Part model, mm, in its own coordinate system. Face numbers are marked on the shaded views. A direction names the side the tool comes from. Coordinates: 2 decimals unless noted, no trailing zeros. Order: outer loops, then holes, each group sorted by start corner. A loop starts at its lowest first (then second) coordinate and runs counter-clockwise, first axis right, second up. Notation, with made-up numbers: (6, -17) - (28, -17) arc R21 ccw to (28, 22) - close; hole circle Ø2 at (18.5, 36). An arc over 180 degrees is marked (long way). Use a Markdown table: item, result. Add a question column.
1) Tool access for the marked faces 1, 2 and 3: list every direction of +Z, -Z, +X, -X, +Y, -Y with a clear straight run to the whole face (end or side of a thin tool).
2) Two-plate mould, pull along X, no slides. Class the marked faces 4, 5 and 6: +X half, -X half, draft (parallel to the pull), parting line (faces both ways), or undercut.
3) Saw through at B-B on x = -22. List the corners of the cut face in (y, z).
4) Drop flat-ended pins along their axis: P1, Ø3, axis at y = 3.5, z = -4, coming from the -X side; P2, Ø3, axis at x = -11.5, y = -0.5, coming from the +Z side; P3, Ø2.5, axis at x = -25, z = -0.5, coming from the +Y side; P4, Ø4, axis at x = -17.5, y = 1, coming from the -Z side. Give the stop position or say it passes through.
5) Saw through at A-A on x = -11.5. List the corners of the cut face in (y, z).
6) Wall check: L1, parallel to X at y = -1, z = -6.5; L2, parallel to Y at x = -14, z = -8.25; L3, parallel to Y at x = -20.25, z = -9. Give the ranges that are in metal, low to high. Write a range as [from, to].
```python
from build123d import *
from build123d.topology import SkipClean

# Parameters (mm, degrees)
BOSS_EXTRUDE1_DEPTH = 1
CUT_EXTRUDE1_DEPTH  = 0.5
BOSS_EXTRUDE2_START = -25
BOSS_EXTRUDE2_DEPTH = 25
BOSS_EXTRUDE3_START = 1
BOSS_EXTRUDE3_DEPTH = 1
SKETCH7_R           = 0.5
BOSS_EXTRUDE4_DEPTH = 22.5
SKETCH10_R          = 0.5
CUT_EXTRUDE4_DEPTH  = 40.5
SKETCH8_W           = 10.868003522
SKETCH8_H           = 5.625
CUT_EXTRUDE2_DEPTH  = 22.5
LPATTERN1_COUNT     = 2
LPATTERN1_PITCH     = 11.25
CUT_EXTRUDE3_START  = -40.5
SKETCH9_R           = 20.473718745
SKETCH9_R_2         = 11.25
CUT_EXTRUDE3_DEPTH  = 40.5
SKETCH11_W          = 6.72531589
SKETCH11_H          = 3.584111804
SKETCH11_W_2        = 7.229090256
SKETCH11_H_2        = 3.619498095
CUT_EXTRUDE5_DEPTH  = 40.5
FILLET1_R           = 3


with BuildPart() as part:
    # Sketch1 → Boss-Extrude1 (new body)
    with BuildSketch(Plane(origin=(0, 0, 0), x_dir=(0, 0, -1), z_dir=(1, 0, 0))):
        with BuildLine():
            Line((0, -2.25), (0, -10.25))
            ThreePointArc((0, -10.25), (10.25, 0), (0, 10.25))
            Line((0, 10.25), (0, 2.25))
            ThreePointArc((0, 2.25), (1.590990258, 1.590990258), (2.25, 0))
            ThreePointArc((2.25, 0), (1.590990258, -1.590990258), (0, -2.25))
        make_face()
    extrude(amount=BOSS_EXTRUDE1_DEPTH)

    # Sketch2 → Cut-Extrude1 (cut)
    with BuildSketch(Plane.ZY):
        with BuildLine():
            ThreePointArc((0, 3.75), (2.651650429, 2.651650429), (3.75, 0))
            ThreePointArc((3.75, 0), (2.651650429, -2.651650429), (0, -3.75))
            Line((0, -3.75), (0, -4.75))
            ThreePointArc((0, -4.75), (3.358757211, -3.358757211), (4.75, 0))
            ThreePointArc((4.75, 0), (3.358757211, 3.358757211), (0, 4.75))
            Line((0, 4.75), (0, 3.75))
        make_face()
        with BuildLine():
            ThreePointArc((0, -3.75), (-3.75, 0), (0, 3.75))
            Line((0, 3.75), (0, 4.75))
            ThreePointArc((0, 4.75), (-4.75, 0), (0, -4.75))
            Line((0, -4.75), (0, -3.75))
        make_face()
        with BuildLine():
            Line((0, 6.75), (0, 5.75))
            ThreePointArc((0, 5.75), (4.065863992, 4.065863992), (5.75, 0))
            ThreePointArc((5.75, 0), (4.065863992, -4.065863992), (0, -5.75))
            Line((0, -5.75), (0, -6.75))
            ThreePointArc((0, -6.75), (4.772970773, -4.772970773), (6.75, 0))
            ThreePointArc((6.75, 0), (4.772970773, 4.772970773), (0, 6.75))
        make_face()
        with BuildLine():
            ThreePointArc((0, -5.75), (-5.75, 0), (0, 5.75))
            Line((0, 5.75), (0, 6.75))
            ThreePointArc((0, 6.75), (-6.75, 0), (0, -6.75))
            Line((0, -6.75), (0, -5.75))
        make_face()
        with BuildLine():
            Line((0, 8.75), (0, 7.75))
            ThreePointArc((0, 7.75), (5.480077554, 5.480077554), (7.75, 0))
            ThreePointArc((7.75, 0), (5.480077554, -5.480077554), (0, -7.75))
            Line((0, -7.75), (0, -8.75))
            ThreePointArc((0, -8.75), (6.187184335, -6.187184335), (8.75, 0))
            ThreePointArc((8.75, 0), (6.187184335, 6.187184335), (0, 8.75))
        make_face()
        with BuildLine():
            ThreePointArc((0, -7.75), (-7.75, 0), (0, 7.75))
            Line((0, 7.75), (0, 8.75))
            ThreePointArc((0, 8.75), (-8.75, 0), (0, -8.75))
            Line((0, -8.75), (0, -7.75))
        make_face()
    extrude(amount=-CUT_EXTRUDE1_DEPTH, mode=Mode.SUBTRACT)

    # Sketch3 → Boss-Extrude2 (add)
    with BuildSketch(Plane(origin=(1, 0, 0), x_dir=(0, 0, -1), z_dir=(1, 0, 0)).offset(BOSS_EXTRUDE2_START)):
        with BuildLine():
            Line((0, -10.25), (0, -11.25))
            ThreePointArc((0, -11.25), (11.25, 0), (0, 11.25))
            Line((0, 11.25), (0, 10.25))
            ThreePointArc((0, 10.25), (10.25, 0), (0, -10.25))
        make_face()
    extrude(amount=BOSS_EXTRUDE2_DEPTH)

    # Sketch6 → Boss-Extrude3 (add)
    with BuildSketch(Plane.ZY.offset(24).offset(BOSS_EXTRUDE3_START)):
        with BuildLine():
            Line((0, 11.25), (0, -11.25))
            ThreePointArc((0, -11.25), (-11.25, 0), (0, 11.25))
        make_face()
    extrude(amount=-BOSS_EXTRUDE3_DEPTH)

    # Sketch7 → Boss-Extrude4 (add)
    with SkipClean():  # the faces are left unmerged after this step: merging them gives an invalid solid
        with BuildSketch(Plane(origin=(0, 11.25, 0), x_dir=(1, 0, 0), z_dir=(0, 1, 0))):
            with BuildLine():
                Line((-23.585786438, 0), (-25, 1.414213562))
                Line((-25, 1.414213562), (-25.707106781, 0.707106781))
                ThreePointArc((-25.707106781, 0.707106781), (-25.707106781, -0.707106781), (-24.292893219, -0.707106781))
                Line((-24.292893219, -0.707106781), (-23.585786438, 0))
            make_face()
            with Locations(Location((-25, 0, 0), (0, 0, 270))):
                Circle(SKETCH7_R, mode=Mode.SUBTRACT)
        extrude(amount=-BOSS_EXTRUDE4_DEPTH)

    # Sketch10 → Cut-Extrude4 (cut)
    with BuildSketch(Plane(origin=(0, 11.25, 0), x_dir=(1, 0, 0), z_dir=(0, 1, 0))):
        with Locations(Location((-25, 0, 0), (0, 0, 270))):
            Circle(SKETCH10_R)
    extrude(amount=-CUT_EXTRUDE4_DEPTH, mode=Mode.SUBTRACT)

    # Sketch8 → Cut-Extrude2 (cut)
    with BuildSketch(Plane(origin=(-11.792893219, 0, -11.792893219), x_dir=(0.7071067811865439, 0, -0.7071067811865511), z_dir=(0.7071067811865511, 0, 0.7071067811865439))):
        with Locations((-22.111671291, 8.4375)):
            Rectangle(SKETCH8_W, SKETCH8_H)
    cut_extrude2 = extrude(amount=-CUT_EXTRUDE2_DEPTH, mode=Mode.SUBTRACT)

    # LPattern1: Cut-Extrude2 ×2
    with Locations(*[(0, -i * LPATTERN1_PITCH, 0) for i in range(1, LPATTERN1_COUNT)]):
        add(cut_extrude2, mode=Mode.SUBTRACT)

    # Sketch9 → Cut-Extrude3 (cut)
    with BuildSketch(Plane(origin=(1, 0, 0), x_dir=(0, 0, -1), z_dir=(1, 0, 0)).offset(CUT_EXTRUDE3_START)):
        Circle(SKETCH9_R)
        Circle(SKETCH9_R_2, mode=Mode.SUBTRACT)
    extrude(amount=CUT_EXTRUDE3_DEPTH, mode=Mode.SUBTRACT)

    # Sketch11 → Cut-Extrude5 (cut)
    with BuildSketch(Plane(origin=(-11.792893219, 0, -11.792893219), x_dir=(0.7071067811865434, 0, -0.7071067811865517), z_dir=(0.7071067811865517, 0, 0.7071067811865434))):
        with Locations((-20.040327475, 1.020444098)):
            Rectangle(SKETCH11_W, SKETCH11_H)
        with Locations((-20.292214658, -10.224678683)):
            Rectangle(SKETCH11_W_2, SKETCH11_H_2)
    extrude(amount=-CUT_EXTRUDE5_DEPTH, mode=Mode.SUBTRACT)

    # Fillet1
    # the kernel refuses this fillet: 3 mm, written as the material it adds along each edge
    with BuildSketch(Plane(origin=(-24, 0, 0), x_dir=(0, 0.7697147606602491, 0.6383879598032339), z_dir=(0, -0.6383879598032339, 0.7697147606602491))) as fillet1_piece_1_section:
        with BuildLine():
            CenterArc((10.25 - FILLET1_R, -FILLET1_R), FILLET1_R, 0, 90)
            Line((10.25 - FILLET1_R, 0), (10.25, 0))
            Line((10.25, 0), (10.25, -FILLET1_R))
        make_face()
    fillet1_piece_1 = revolve(axis=Axis((-24, 0, 0), (-1, 0, 0)), revolution_arc=259.343436967, mode=Mode.PRIVATE)
    fillet1_piece_1 = split(fillet1_piece_1, bisect_by=Plane(origin=(-23.150246859, 0, 0), z_dir=(0, 0, -1)), keep=Keep.TOP, mode=Mode.PRIVATE)
    fillet1_piece_1 = split(fillet1_piece_1, bisect_by=Plane(origin=(-28.068140078, 0, -4.482353641), z_dir=(0.7071067811865434, 0, -0.7071067811865517)), keep=Keep.TOP, mode=Mode.PRIVATE)
    add(fillet1_piece_1)


solid = part.part
```
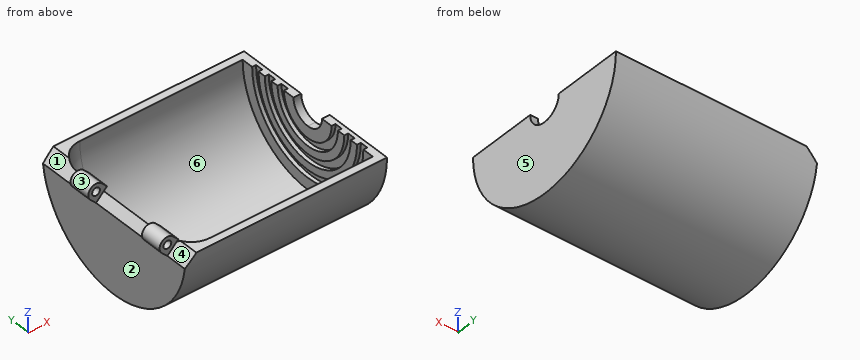
Results are:
| question | item | result |
|---|---|---|
| 1 | face 1 | +Z, -X, +Y |
| 1 | face 2 | -Z, -X, +Y, -Y |
| 1 | face 3 | +Y, -Y |
| 2 | face 4 | -X half |
| 2 | face 5 | +X half |
| 2 | face 6 | undercut |
| 3 | outline | (-11.25, 0) arc R11.25 ccw to (11.25, 0) - (10.08, 0) arc R10.08 cw to (-10.08, 0) - close |
| 4 | P1 | x = -25 |
| 4 | P2 | z = -10.05 |
| 4 | P3 | y = 11.25 |
| 4 | P4 | z = -11.25 |
| 5 | outline | (-11.25, 0) arc R11.25 ccw to (11.25, 0) - (10.25, 0) arc R10.25 cw to (-10.25, 0) - close |
| 6 | L1 | [-25, -24], [0.5, 1] |
| 6 | L2 | [-7.65, -6.08], [6.08, 7.65] |
| 6 | L3 | [-6.75, -4.91], [4.91, 6.75] |
